Source: CAD feature listing. Evaluate the final solid. Frame: model axes, mm. Face numbers are marked on the shaded views. Round coordinates to 2 decimals unless told otherwise and drop trailing zeros. Loops run counter-clockwise (first coordinate to the right, second up) from the corner with the lowest first, then second, coordinate; pieces in that order, holes last. Notation, with made-up numbers: (36, -15.5) - (52, -15.5) arc R30 cw to (52, 17.5) - close; hole circle Ø9 at (21.5, 88). An arc over 180 degrees is marked (long way). Use CSV: the item, a comma, the result in double quotes. Start each with the question number.
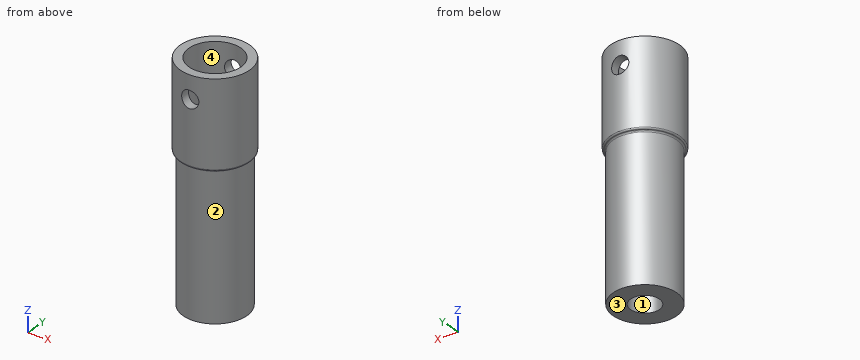
from build123d import *

# Parameters (mm, degrees)
SKETCH1_R               = 12
SKETCH1_R_2             = 9
BOSS_EXTRUDE1_DEPTH     = 30
SKETCH2_R               = 11
BOSS_EXTRUDE2_DEPTH     = 50
SKETCH3_R               = 5
CUT_EXTRUDE1_DEPTH      = 40
CUT_EXTRUDE2_DEPTH      = 53.80151513
CUT_EXTRUDE2_DEPTH_BACK = 53.80151513
SKETCH4_R               = 3
FILLET1_R               = 0.5


with BuildPart() as part:
    # Sketch1 → Boss-Extrude1 (new body)
    with BuildSketch(Plane.XY):
        Circle(SKETCH1_R)
        Circle(SKETCH1_R_2, mode=Mode.SUBTRACT)
    extrude(amount=BOSS_EXTRUDE1_DEPTH)

    # Sketch2 → Boss-Extrude2 (add)
    with BuildSketch(Plane(origin=(0, 0, 0), x_dir=(-1, 0, 0), z_dir=(0, 0, -1))):
        Circle(SKETCH2_R)
    extrude(amount=BOSS_EXTRUDE2_DEPTH)

    # Sketch3 → Cut-Extrude1 (cut)
    with BuildSketch(Plane(origin=(0, 0, -50), x_dir=(-1, 0, 0), z_dir=(0, 0, -1))):
        Circle(SKETCH3_R)
    extrude(amount=-CUT_EXTRUDE1_DEPTH, mode=Mode.SUBTRACT)

    # Sketch4 → Cut-Extrude2 (cut, two sides: drawn at the far end of the back side and taken through both)
    with BuildSketch(Plane(origin=(0, 0, 0), x_dir=(1, 0, 0), z_dir=(0, 1, 0)).offset(-CUT_EXTRUDE2_DEPTH_BACK)):
        with Locations(Location((0, -22, 0), (0, 0, 270))):
            Circle(SKETCH4_R)
    extrude(amount=CUT_EXTRUDE2_DEPTH + CUT_EXTRUDE2_DEPTH_BACK, mode=Mode.SUBTRACT)

    # Fillet1
    fillet1_edges = [part.edges().sort_by_distance(p)[0] for p in [
        (-12, 0, 0),
        (11, 0, 0),
    ]]
    fillet(fillet1_edges, radius=FILLET1_R - 0.0001)  # a hair under: the kernel refuses the full size


solid = part.part
1. Line query: line 1 along Z through (x, y) = (0, -10.85); line 2 along Z through (x, y) = (3.5, -7); line 3 along Z through (x, y) = (6.25, 9.5). Output: solid intervals per line, ascending.
2. Section query D-D on z = -11. Return the cut outline in (x, y).
3. Mould query, pull axis Y, two halves, no side actions, for the marked faces 1, 2, 3 and 4. Classes: +Y half, -Y half, draft (parallel to the pull), parting line (faces both ways), or undercut.
4. Section query B-B on z = 22. Return the cut outline in (x, y).
5. Contact query for flat-ended pins moving along their axis: P1, Ø4, axis at y = -6.5, z = 15, coming from the -X side; P2, Ø3, axis at x = 7.5, z = 17.5, coming from the -Y side; P3, Ø1.5, axis at y = -5, z = 17.5, coming from the -X side. Output: stop coordinate, or through.
6. Section query A-A on x = 0. Give the number of separate pieces and of enclosed holes in the cut face, and give its area (3 significant figures).
Values:
1,line 1,"z = -50 to 19, 25 to 30"
1,line 2,"z = -50 to 0"
1,line 3,"z = -0.02 to 30"
2,outline,"circle Ø22 at (0, 0); hole circle Ø10 at (0, 0)"
3,face 1,"undercut"
3,face 2,"parting line"
3,face 3,"draft"
3,face 4,"undercut"
4,outline,"(-3, -11.62) - (-3, -8.49) arc R9 cw to (-3, 8.49) - (-3, 11.62) arc R12 ccw to start; (3, -11.62) arc R12 ccw to (3, 11.62) - (3, 8.49) arc R9 cw to (3, -8.49) - close"
5,P1,"stops at x = -11.12"
5,P2,"stops at y = -10.39"
5,P3,"stops at x = -11.22"
6,separate pieces,"3"
6,enclosed holes,"0"
6,area,"844 mm^2"
